from build123d import *

# Parameters (mm, degrees)
SKETCH1_W           = 497
SKETCH1_H           = 176.5
SKETCH1_R           = 2.5
BOSS_EXTRUDE1_DEPTH = 18
SKETCH2_R           = 5
CUT_EXTRUDE1_DEPTH  = 13


with BuildPart() as part:
    # Sketch1 → Boss-Extrude1 (new body)
    with BuildSketch(Plane.XY):
        with Locations((0, -482.25)):
            Rectangle(SKETCH1_W, SKETCH1_H)
        with Locations((64, -482.25)):
            Circle(SKETCH1_R, mode=Mode.SUBTRACT)
        with Locations((-64, -482.25)):
            Circle(SKETCH1_R, mode=Mode.SUBTRACT)
    extrude(amount=BOSS_EXTRUDE1_DEPTH)

    # Sketch2 → Cut-Extrude1 (cut)
    with BuildSketch(Plane(origin=(0, 0, 0), x_dir=(-1, 0, 0), z_dir=(0, 0, -1))):
        with Locations((224, -514)):
            Circle(SKETCH2_R)
        with Locations((-224, -514)):
            Circle(SKETCH2_R)
        with Locations((224, -450)):
            Circle(SKETCH2_R)
        with Locations((-224, -450)):
            Circle(SKETCH2_R)
    extrude(amount=-CUT_EXTRUDE1_DEPTH, mode=Mode.SUBTRACT)


solid = part.part
For this review, take the finished solid that the model builds, in its own axes (mm). A direction names the side the tool comes from. Coordinates: 2 decimals unless noted, no trailing zeros. Loops run counter-clockwise (first coordinate to the right, second up) from the corner with the lowest first, then second, coordinate; pieces in that order, holes last. Notation, with made-up numbers: (-13.5, 15.25) - (13.5, 15.25) arc R17 ccw to (13.5, 22.25) - close; hole circle Ø11 at (78.25, 78.5). An arc over 180 degrees is marked (long way). Return JSON: item names as keys, results as strings.
Item 1: Insertion check: pin 1 (11 mm diameter, centred on x = -223.5, y = -511.5, fed in from -Z); pin 2 (3 mm diameter, centred on x = 222, y = -448.5, fed in from -Z). Each pin has a flat end and moves straight along its axis. Give the tip position at first contact, or say it passes through.
Determined:
{"pin 1": "stops at z = 0", "pin 2": "stops at z = 13"}
Item 2: Take a section at B-B (x = -224). Give the boundary of the cut face in (y, z).
Determined:
{"outline": "(-570.5, 0) - (-519, 0) - (-519, 13) - (-509, 13) - (-509, 0) - (-455, 0) - (-455, 13) - (-445, 13) - (-445, 0) - (-394, 0) - (-394, 18) - (-570.5, 18) - close"}
Item 3: Mouldability with a two-part tool opening along X and no side actions: class faces 1 (the flat face through (-248.5, -483, 9)), 2 (the flat face through (-3, -394, 9)), 3 (the flat face through (-224, -514, 13)) as pulls with the +X half, pulls with the -X half, needs draft (parallel to the pull), parting line crosses it, or undercut.
Determined:
{"face 1": "pulls with the -X half", "face 2": "needs draft", "face 3": "undercut"}
Item 4: Take a section at A-A (y = -450). Give the boundary of the cut face in (x, z).
Determined:
{"outline": "(-248.5, 0) - (-229, 0) - (-229, 13) - (-219, 13) - (-219, 0) - (219, 0) - (219, 13) - (229, 13) - (229, 0) - (248.5, 0) - (248.5, 18) - (-248.5, 18) - close"}
Item 5: For faces 4 (the cylindrical face through (-227, -510, 6)), 5 (the flat face through (-3, -481, 18)), list the 3-axis set-ups (+Z, -Z, +X, -X, +Y, -Y) from which the entire face can be reached by the end or side of a thin tool; tool diameter is ignored.
Determined:
{"face 4": "-Z", "face 5": "+Z, +X, -X, +Y, -Y"}
Item 6: For line 1 (X direction, y = -450, z = 3.5); line 2 (Y direction, x = -224, z = 3.5); line 3 (X direction, y = -451, z = 5.25), list the stretches that pass through material, from the lowest coordinate up.
Determined:
{"line 1": "x = -248.5 to -229, -219 to 219, 229 to 248.5", "line 2": "y = -570.5 to -519, -509 to -455, -445 to -394", "line 3": "x = -248.5 to -228.9, -219.1 to 219.1, 228.9 to 248.5"}
